Check sheet for the modelled part. Datum: model origin and axes. Units: mm. A direction names the side the tool comes from. Give positions to 0.01 mm unless a question says otherwise; leave off trailing zeros. Order: outer loops, then holes, each group sorted by start corner. A loop starts at its lowest first (then second) coordinate and runs counter-clockwise, first axis right, second up. Notation, with made-up numbers: (-30, 25) -> (-8, 25) arc R8 ccw to (-8, 37) -> close; hole circle Ø4 at (10, 8.5). An arc over 180 degrees is marked (long way). One line per question, with ' | ' between items.
```python
from build123d import *

# Parameters (mm, degrees)
F0_W     = 45
F0_H     = 45
F0_R     = 2.5
F1_DEPTH = 30
F0_W_2   = 50.2
F0_H_2   = 50.2
F2_DEPTH = 2
F3_T     = -2
F4_R     = 5
F5_SIZE  = 1.5


with BuildPart() as f1:
    # F0 (on Top) → F1 (new body)
    with BuildSketch(Plane.XY):
        Rectangle(F0_W, F0_H)
        Circle(F0_R, mode=Mode.SUBTRACT)
    extrude(amount=F1_DEPTH)

    # F0 (on Top) → F2 (join)
    with BuildSketch(Plane.XY):
        Rectangle(F0_W_2, F0_H_2)
        Rectangle(F0_W, F0_H, mode=Mode.SUBTRACT)
    extrude(amount=F2_DEPTH)

    # F3
    f3_openings = [f1.faces().sort_by_distance(p)[0] for p in [
        (0, 21.863604, 30),
        (-2.5, 0, 15),
    ]]
    offset(amount=F3_T, openings=f3_openings, kind=Kind.INTERSECTION)

    # F4
    f4_edges = [f1.edges().sort_by_distance(p)[0] for p in [
        (-22.5, -22.5, 16),
        (22.5, -22.5, 16),
        (22.5, 22.5, 16),
        (-22.5, 22.5, 16),
        (20.5, 20.5, 16),
        (-20.5, 20.5, 16),
        (-20.5, -20.5, 16),
        (20.5, -20.5, 16),
    ]]
    fillet(f4_edges, radius=F4_R)

    # F5
    f5_edges = [f1.edges().sort_by_distance(p)[0] for p in [
        (25.1, 25.1, 1),
        (25.1, -25.1, 1),
        (-25.1, 25.1, 1),
        (-25.1, -25.1, 1),
    ]]
    chamfer(f5_edges, length=F5_SIZE)


solid = f1.part
```
Q1. Depth check by flat-ended pin: pin 1 Ø1 at (x, z) = (2, 22.5) entering from -Y; pin 2 Ø20.5 at (x, y) = (-7.5, -1) entering from +Z; pin 3 Ø1 at (x, y) = (12, -17.5) entering from -Z; pin 4 Ø14 at (y, z) = (-3, 20) entering from -X. Enter the tip coordinate at first touch or a pass-through.
Result sheet:
pin 1: stops at y = -22.5 | pin 2: stops at z = 2 | pin 3: stops at z = 0 | pin 4: stops at x = -22.5
Q2. Mould release check, pull along Y, two halves, no side actions. Record for faces 1 (the face through (0, 20.5, 16)), 2 (the face through (0, -25.1, 1)), 3 (the face through (25.1, 0, 1)): pulls with the +Y half, pulls with the -Y half, needs draft (parallel to the pull), parting line crosses it, or undercut.
Result sheet:
face 1: undercut | face 2: pulls with the -Y half | face 3: needs draft
Q3. Section check C-C (x = -6). Enter the section's corners in (y, z), and give its area (3 significant figures).
Result sheet:
outline: (-25.1, 0) -> (25.1, 0) -> (25.1, 2) -> (22.5, 2) -> (22.5, 30) -> (20.5, 30) -> (20.5, 2) -> (-20.5, 2) -> (-20.5, 30) -> (-22.5, 30) -> (-22.5, 2) -> (-25.1, 2) -> close | area: 212 mm2
Q4. Access from +Z, -Z, +X, -X, +Y, -Y to the whole of each face (thin tool, end or side, straight path). Record for faces 4 (the face through (21.07, 21, 16.2)), 5 (the face through (22.5, 0, 16)), 6 (the face through (20.5, 0, 16)).
Result sheet:
face 4: +Z, +X, +Y | face 5: +Z, +X, +Y, -Y | face 6: +Z
Q5. Section check B-B (z = 22.5). Enter the section's corners in (x, y), and give its area (3 significant figures).
Result sheet:
outline: (-22.5, -17.5) arc R5 ccw to (-17.5, -22.5) -> (17.5, -22.5) arc R5 ccw to (22.5, -17.5) -> (22.5, 17.5) arc R5 ccw to (17.5, 22.5) -> (-17.5, 22.5) arc R5 ccw to (-22.5, 17.5) -> close; hole (-20.5, -15.5) arc R5 ccw to (-15.5, -20.5) -> (15.5, -20.5) arc R5 ccw to (20.5, -15.5) -> (20.5, 15.5) arc R5 ccw to (15.5, 20.5) -> (-15.5, 20.5) arc R5 ccw to (-20.5, 15.5) -> close | area: 344 mm2
Q6. Thickness scan on line 1 (Y direction, x = 13.5, z = 19.5); line 2 (X direction, y = 0, z = 0.75). Record the ranges inside material, lowest first.
Result sheet:
line 1: y = -22.5 to -20.5, 20.5 to 22.5 | line 2: x = -25.1 to -2.5, 2.5 to 25.1
Q7. Section check A-A (y = 0). Enter the section's corners in (x, z), and give its area (3 significant figures).
Result sheet:
outline: (-25.1, 0) -> (-2.5, 0) -> (-2.5, 2) -> (-20.5, 2) -> (-20.5, 30) -> (-22.5, 30) -> (-22.5, 2) -> (-25.1, 2) -> close; (2.5, 0) -> (25.1, 0) -> (25.1, 2) -> (22.5, 2) -> (22.5, 30) -> (20.5, 30) -> (20.5, 2) -> (2.5, 2) -> close | area: 202 mm2
